from build123d import *

# Parameters (mm, degrees)
F1_DEPTH = 5
F3_DEPTH = 8
F4_R     = 1
F5_ANGLE = 180


with BuildPart() as f1:
    # F0 (on Top) → F1 (new body)
    with BuildSketch(Plane.XY):
        with BuildLine():
            Line((-4.734272, 0), (-2.367136, 4.1))
            Line((-2.367136, 4.1), (2.367136, 4.1))
            Line((2.367136, 4.1), (2.800149, 3.35))
            Line((2.800149, 3.35), (5.841911, 3.35))
            ThreePointArc((5.841911, 3.35), (-6.734272, 0), (5.841911, -3.35))
            Line((5.841911, -3.35), (2.800149, -3.35))
            Line((2.800149, -3.35), (2.367136, -4.1))
            Line((2.367136, -4.1), (-2.367136, -4.1))
            Line((-2.367136, -4.1), (-4.734272, 0))
        make_face()
    extrude(amount=-F1_DEPTH)

    # F2 (on Top) → F3 (join)
    with BuildSketch(Plane.XY):
        with BuildLine():
            Line((5.841911, -3.35), (3.35, -3.35))
            Line((3.35, -3.35), (-3.35, -3.35))
            Line((-3.35, -3.35), (-3.35, 3.35))
            Line((-3.35, 3.35), (3.35, 3.35))
            Line((3.35, 3.35), (5.841911, 3.35))
            ThreePointArc((5.841911, 3.35), (-6.734272, 0), (5.841911, -3.35))
        make_face()
    extrude(amount=F3_DEPTH)

    # F4
    f4_edges = [f1.edges().sort_by_distance(p)[0] for p in [
        (5.841911, 3.35, 1.5),
        (5.841911, -3.35, 1.5),
    ]]
    fillet(f4_edges, radius=F4_R)


with BuildPart() as f1_1:
    # F5: moved
    add(f1.part.rotate(Axis((-3.35, 0, 8), (0, -1, 0)), F5_ANGLE))


solid = f1_1.part
Could you check a few things on this model? Use its own coordinates, in mm. A direction names the side the tool comes from. Coordinates: 2 decimals unless noted, no trailing zeros. Order: outer loops, then holes, each group sorted by start corner. A loop starts at its lowest first (then second) coordinate and runs counter-clockwise, first axis right, second up.
Q1. Suppose I cut it at D-D on x = -8.25. Please give me the cut outline in (y, z), and give its area (3 significant figures).
Q2. Thinking about a two-plate mould opening in Y: for faces 1 (the flat face through (-3.13, 2.02, 18.46)), 2 (the cylindrical face through (0.03, 0.21, 14.59)), 3 (the flat face through (-7, 3.35, 12)), 4 (the flat face through (-3, 0, 8)), which applies, released by +Y, released by -Y, zero draft, split by the parting line, or undercut?
Q3. Suppose I cut it at A-A on x = -6.7. Please give me the cut outline in (y, z).
Q4. Please list where these lines run through material, in increasing order: L1, parallel to Y at x = -6.5, z = 20.5; L2, parallel to Y at x = -6.5, z = 11.75; L3, parallel to Z at x = -3.5, y = -3.25.
Q5. Suppose I cut it at C-C on y = 2. Please give me the cut outline in (x, z), and give its area (3 significant figures).
Q6. Which directions (+Z, -Z, +X, -X, +Y, -Y) give clear straight access to the entire face, cutting with the end or side of a thin tool? Please do faces 5 (the flat face through (-1.8, 0.1, 21)), 6 (the cylindrical face through (-11.37, 3.99, 14.59)), 7 (the flat face through (-3, 0, 16)), 8 (the flat face through (-3.35, 0, 12)), 9 (the flat face through (-7, -4.1, 18)).
Q7. Suppose I cut it at B-B on z = 12. Please give me the cut outline in (x, y), and give its area (3 significant figures).
Q8. Will these pins go through, and if not, where does the flat tip stop? pin 1 (1.5 mm diameter, centred on y = 1, z = 17.5, fed in from +X); pin 2 (2 mm diameter, centred on x = -9, z = 15.5, fed in from -Y); pin 3 (0.8 mm diameter, centred on x = -7.5, y = -3.5, fed in from +Z).
Answer:
1. outline: (-6.55, 8) - (-3.35, 8) - (-3.35, 16) - (-4.1, 16) - (-4.1, 21) - (-6.55, 21) - close; (3.35, 8) - (6.55, 8) - (6.55, 21) - (4.1, 21) - (4.1, 16) - (3.35, 16) - close
1. area: 75.8 mm2
2. face 1: undercut
2. face 2: split by the parting line
2. face 3: undercut
2. face 4: zero draft
3. outline: (-6.73, 8) - (-3.35, 8) - (-3.35, 16) - (-4.1, 16) - (-4.1, 21) - (-6.73, 21) - close; (3.35, 8) - (6.73, 8) - (6.73, 21) - (4.1, 21) - (4.1, 16) - (3.35, 16) - close
4. L1: y = -6.73 to -4.1, 4.1 to 6.73
4. L2: y = -6.73 to -3.35, 3.35 to 6.73
4. L3: z = 16 to 21
5. outline: (-3.35, 8) - (-0.27, 8) - (-0.27, 21) - (-3.12, 21) - (-3.12, 16) - (-3.35, 16) - close
5. area: 38.9 mm2
6. face 5: +Z, +X, -X, +Y, -Y
6. face 6: +Z, -Z, -X
6. face 7: +Z, -X
6. face 8: -Z, -X
6. face 9: +Z
7. outline: (-11.09, -5.11) arc R6.73 ccw (long way) to (-11.09, 5.11) arc R1 ccw to (-10.44, 3.35) - (-3.35, 3.35) - (-3.35, -3.35) - (-10.44, -3.35) arc R1 ccw to start
7. area: 74.6 mm2
8. pin 1: stops at x = 0.03
8. pin 2: stops at y = -6.61
8. pin 3: stops at z = 16
